Study the drawing (mm; zero at the part's minimum x, y, z) and answer. A direction names the side the tool comes from. Round coordinates to 2 decimals unless told otherwise and drop trailing zeros. Write each loop counter-clockwise with the first axis right and the second up, starting at its lowest first coordinate (ties: lowest second). Pieces come first, ordered by that corner, then holes.
(1) A cutting plane is placed at B-B, the plane z = 2. Give the vertices of the cut face in (x, y).
(2) Each of these flat-tipped pins is pushed along its axis until it touches: pin 1 Ø3 at (x, z) = (6.5, 2.5) entering from -Y; pin 2 Ø1.6 at (x, y) = (4.5, 0.5) entering from -Z. Where does it stop, or does it pass through?
(3) A cutting plane is placed at C-C, the plane y = 12.75. Give the vertices of the cut face in (x, z).
(4) A cutting plane is placed at A-A, the plane x = 6. Give the vertices of the cut face in (y, z), and give its area (3 significant figures).
(5) For the marked faces 1, 2 and 3, determine the directions among +Z, -Z, +X, -X, +Y, -Y from which every point of the face is accessible in a straight line to the end or side of a thin tool.
(6) Find the intervals of material crossed by probe 1 along Y at (x, z) = (4, 2.25); probe 2 along Z at (x, y) = (2.5, 13), in increasing order.
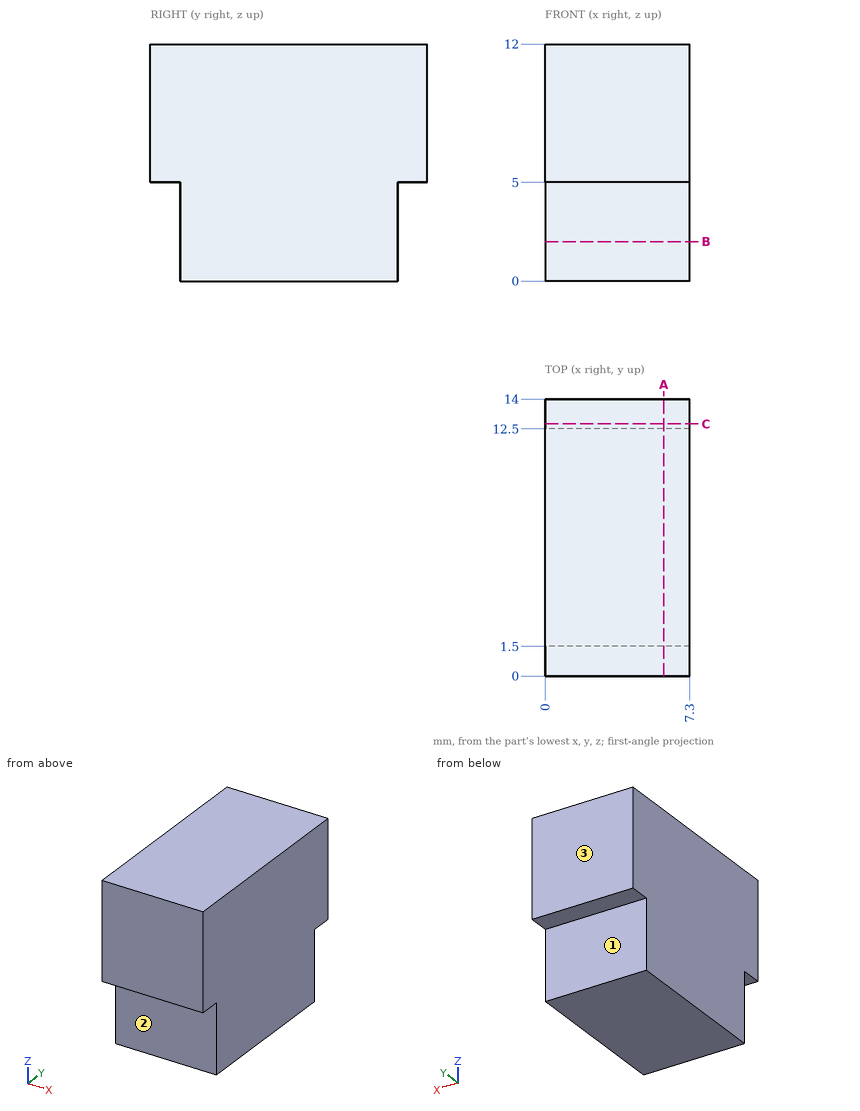
Solutions:
1. outline: (0, 1.5) - (7.3, 1.5) - (7.3, 12.5) - (0, 12.5) - close
2. pin 1: stops at y = 1.5
2. pin 2: stops at z = 5
3. outline: (0, 5) - (7.3, 5) - (7.3, 12) - (0, 12) - close
4. outline: (0, 5) - (1.5, 5) - (1.5, 0) - (12.5, 0) - (12.5, 5) - (14, 5) - (14, 12) - (0, 12) - close
4. area: 153 mm2
5. face 1: -Z, +X, -X, +Y
5. face 2: -Z, +X, -X, -Y
5. face 3: +Z, -Z, +X, -X, +Y
6. probe 1: y = 1.5 to 12.5
6. probe 2: z = 5 to 12
